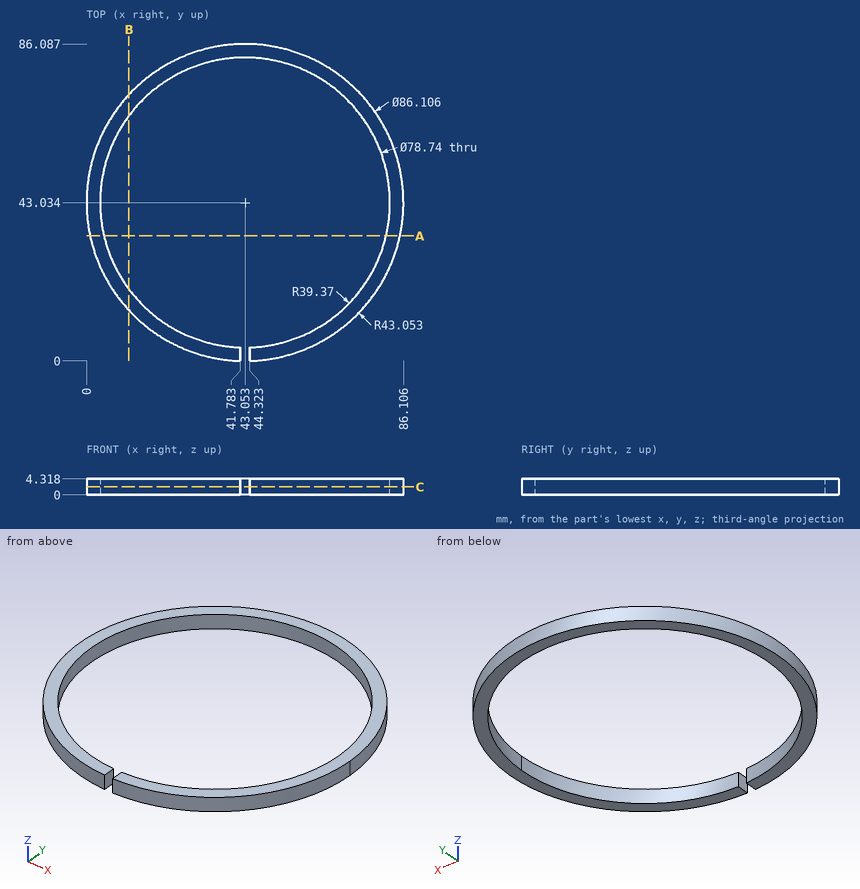
Study the drawing (mm; zero at the part's minimum x, y, z) and answer. Coordinates: 2 decimals unless noted, no trailing zeros. Write each loop counter-clockwise with the first axis right and the second up, starting at its lowest first coordinate (ties: lowest second). Pieces come first, ordered by that corner, then holes. Notation, with made-up numbers: (64, 72) - (76, 72) arc R20 ccw to (76, 79) - close; hole circle Ø11 at (-17.75, 71). An arc over 180 degrees is marked (long way). Answer as a JSON object with one key per item and string values. Group by question number.
1. A cutting plane is placed at B-B (x = 11.5). Determine the outline of the cut face in (y, z) (1 decimal).
2. Consider L1, parallel to X at y = 68, z = 0.4 (1 decimal); L2, parallel to X at y = 73, z = 2.8 (1 decimal); L3, parallel to Y at x = 34.5, z = 0.55 (1 decimal). Determine where each line is inside the solid, lowest interval first. Write a range as [from, to].
3. A cutting plane is placed at C-C (z = 2.15). Determine the outline of the cut face in (x, y) (1 decimal).
4. A cutting plane is placed at A-A (y = 34). Determine the outline of the cut face in (x, z).
5. Each of these flat-tipped pins is pushed along its axis until it touches: P1, Ø2, axis at y = 45, z = 1, coming from the +X side (3 decimals); P2, Ø2, axis at y = 52, z = 4, coming from the -X side. Where does it stop, or does it pass through?
Worked out:
{
 "1": {"outline": "(13.7, 0) - (19.5, 0) - (19.5, 4.3) - (13.7, 4.3) - close; (66.6, 0) - (72.3, 0) - (72.3, 4.3) - (66.6, 4.3) - close"},
 "2": {"L1": "x = [8, 12.6], [73.5, 78.1]", "L2": "x = [12.1, 17.5], [68.6, 74]", "L3": "y = [0.8, 4.6], [81.5, 85.2]"},
 "3": {"outline": "(41.8, 0) - (41.8, 3.7) arc R39.4 cw (long way) to (44.3, 3.7) - (44.3, 0) arc R43.1 ccw (long way) to start"},
 "4": {"outline": "(0.96, 0) - (4.73, 0) - (4.73, 4.32) - (0.96, 4.32) - close; (81.37, 0) - (85.15, 0) - (85.15, 4.32) - (81.37, 4.32) - close"},
 "5": {"P1": "stops at x = 86.095", "P2": "stops at x = 0.74"}
}
